Here's how the part is built. I have some questions about the finished solid (model axes, mm). A direction names the side the tool comes from. Give positions to 0.01 mm unless a question says otherwise; leave off trailing zeros. Order: outer loops, then holes, each group sorted by start corner. A loop starts at its lowest first (then second) coordinate and runs counter-clockwise, first axis right, second up. Notation, with made-up numbers: M -24,82 L -7,82 A16 ccw -7,95 Z; hole C 72,64.25 d10. An arc over 180 degrees is marked long. Use one line per item in the form item = value.
from build123d import *

# Parameters (mm, degrees)
SKETCH1_R           = 3
SKETCH1_R_2         = 3.2
SKETCH1_R_3         = 1.75
BOSS_EXTRUDE1_DEPTH = 4
SKETCH1_4_R         = 3
SKETCH1_4_R_2       = 3.2
BOSS_EXTRUDE2_DEPTH = 32


with BuildPart() as part:
    # Sketch1 → Boss-Extrude1 (new body)
    with BuildSketch(Plane.XY):
        with Locations((0, -30)):
            Circle(SKETCH1_R)
        with BuildLine():
            Line((-5.2, 0), (-5.144370275, -0.758587154))
            ThreePointArc((-5.144370275, -0.758587154), (0, -5.2), (5.144370275, -0.758587154))
            Line((5.144370275, -0.758587154), (5.2, 0))
            ThreePointArc((5.2, 0), (0, 5.2), (-5.2, 0))
        make_face()
        Circle(SKETCH1_R_2, mode=Mode.SUBTRACT)
        with BuildLine():
            Line((-5.144370275, -0.758587154), (-3, -30))
            ThreePointArc((-3, -30), (0, -27), (3, -30))
            Line((3, -30), (5.144370275, -0.758587154))
            ThreePointArc((5.144370275, -0.758587154), (0, -5.2), (-5.144370275, -0.758587154))
        make_face()
        with Locations((0, -14.430389534)):
            Circle(SKETCH1_R_3, mode=Mode.SUBTRACT)
    extrude(amount=BOSS_EXTRUDE1_DEPTH)

    # Sketch1_4 → Boss-Extrude2 (add)
    with BuildSketch(Plane.XY):
        with Locations((0, -30)):
            Circle(SKETCH1_4_R)
        with BuildLine():
            Line((-5.2, 0), (-5.144370275, -0.758587154))
            ThreePointArc((-5.144370275, -0.758587154), (0, -5.2), (5.144370275, -0.758587154))
            Line((5.144370275, -0.758587154), (5.2, 0))
            ThreePointArc((5.2, 0), (0, 5.2), (-5.2, 0))
        make_face()
        Circle(SKETCH1_4_R_2, mode=Mode.SUBTRACT)
    extrude(amount=-BOSS_EXTRUDE2_DEPTH)


solid = part.part
Q1. I want a section at B-B on z = -9. Write out the boundary of the cut face in (x, y), then the cut area to 3 significant figures.
Found:
outline = M -5.2,0 L -5.14,-0.76 A5.2 ccw 5.14,-0.76 L 5.2,0 A5.2 ccw Z; C 0,-30 d6; hole C 0,0 d6.4
area = 81.0 mm²
Q2. Thinking about a two-plate mould opening in Y: for faces 3 (the face through (0, -30, -32)), 4 (the face through (-0.38, -16.14, 1.97)), 5 (the face through (0.1, 5.2, -14.3)), which applies, +Y half, -Y half, draft (parallel to the pull), parting line (faces both ways), or undercut?
Found:
face_3 = draft
face_4 = undercut
face_5 = +Y half
Q3. I need wall thicknesses on L1, parallel to Y at x = 0, z = -22; L2, parallel to Y at x = 0, z = 2.55; L3, parallel to Z at x = 3, y = -23. Which ranges of each line are inside material? Lowest first, please.
Found:
L1 = -33 to -27, -5.2 to -3.2, 3.2 to 5.2
L2 = -33 to -16.18, -12.68 to -3.2, 3.2 to 5.2
L3 = 0 to 4
Q4. I want a section at A-A on x = 0. Write out the boundary of the cut face in (y, z).
Found:
outline = M -33,-32 L -27,-32 L -27,0 L -16.18,0 L -16.18,4 L -33,4 Z; M -12.68,0 L -5.2,0 L -5.2,-32 L -3.2,-32 L -3.2,4 L -12.68,4 Z; M 3.2,-32 L 5.2,-32 L 5.2,4 L 3.2,4 Z
Q5. I'm going to push a flat-ended pin straight in: pin 1 Ø4 at (x, y) = (0, -14.43) entering from -Z. Where does the tip first touch, or does it pass through?
Found:
pin_1 = 0
Q6. I want a section at C-C on y = 2.5. Write out the boundary of the cut face in (x, z), then the cut area to 3 significant figures.
Found:
outline = M -4.56,-32 L -2,-32 L -2,4 L -4.56,4 Z; M 2,-32 L 4.56,-32 L 4.56,4 L 2,4 Z
area = 184 mm²
Q7. On a 3-axis mill with a long thin cutter (end or side, diameter ignored), from which of +Z, -Z, +X, -X, +Y, -Y can I reach the whole of each face in a straight line? I mean faces 1 (the face through (-0.65, -32.93, -13.75)), 2 (the face through (-0.1, -3.4, -32)). Say none if no direction works.
Found:
face_1 = -Z
face_2 = -Z, +X, -X, +Y, -Y
Q8. I want a section at D-D on x = 2.5. Write out the boundary of the cut face in (y, z), then the cut area to 3 significant figures.
Found:
outline = M -31.66,-32 L -28.34,-32 L -28.34,0 L -4.56,0 L -4.56,-32 L -2,-32 L -2,4 L -31.66,4 Z; M 2,-32 L 4.56,-32 L 4.56,4 L 2,4 Z
area = 399 mm²
